Here's how the part is built. I have some questions about the finished solid (model axes, mm). Coordinates: 2 decimals unless noted, no trailing zeros. Write each loop counter-clockwise with the first axis right and the second up, starting at its lowest first coordinate (ties: lowest second). Pieces come first, ordered by that corner, then holes.
```python
from build123d import *

# Parameters (mm, degrees)
F0_W     = 53
F0_H     = 53
F0_R     = 1
F0_R_2   = 25.5
F1_DEPTH = 2
F2_SIZE  = 1.99999
F3_R     = 1


# Not quite as in the source:
# - a fillet or chamfer is up to 0.001 mm smaller than in the source, because OpenCascade refuses the exact size


with BuildPart() as f1:
    # F0 (on Top) → F1 (new body)
    with BuildSketch(Plane.XY):
        Rectangle(F0_W, F0_H)
        with Locations((-21.2132034356, -21.2132034356)):
            Circle(F0_R, mode=Mode.SUBTRACT)
        with Locations((21.2132034356, -21.2132034356)):
            Circle(F0_R, mode=Mode.SUBTRACT)
        with Locations((-21.2132034356, 21.2132034356)):
            Circle(F0_R, mode=Mode.SUBTRACT)
        Circle(F0_R_2, mode=Mode.SUBTRACT)
        with Locations((21.2132034356, 21.2132034356)):
            Circle(F0_R, mode=Mode.SUBTRACT)
    extrude(amount=F1_DEPTH)

    # F2 (size 2 in the source; OpenCascade refuses exactly that, so slightly less here)
    f2_edges = [f1.edges().sort_by_distance(p)[0] for p in [
        (-22.213203, 21.213203, 2),
        (20.213203, 21.213203, 2),
        (20.213203, -21.213203, 2),
        (-22.213203, -21.213203, 2),
    ]]
    chamfer(f2_edges, length=F2_SIZE)

    # F3
    f3_edges = [f1.edges().sort_by_distance(p)[0] for p in [
        (26.5, -26.5, 1),
        (26.5, 26.5, 1),
        (-26.5, -26.5, 1),
        (-26.5, 26.5, 1),
    ]]
    fillet(f3_edges, radius=F3_R)


solid = f1.part
```
1) We'd pull the mould along X, two halves only. Please class faces 1 (the face through (-5.5, -24.9, 1)), 2 (the face through (-26.5, 0, 1)), 3 (the face through (0, 26.5, 1)): pulls with the +X half, pulls with the -X half, needs draft (parallel to the pull), parting line crosses it, or undercut.
Values follow:
face 1: undercut
face 2: pulls with the -X half
face 3: needs draft
2) Imagine slicing it at C-C on z = 0.8. Please give me the cut outline in (x, y), then the cut area to 3 significant figures.
Values follow:
outline: (-26.5, -25.5) arc R1 ccw to (-25.5, -26.5) - (25.5, -26.5) arc R1 ccw to (26.5, -25.5) - (26.5, 25.5) arc R1 ccw to (25.5, 26.5) - (-25.5, 26.5) arc R1 ccw to (-26.5, 25.5) - close; hole circle Ø51 at (0, 0); hole circle Ø3.6 at (-21.21, -21.21); hole circle Ø3.6 at (-21.21, 21.21); hole circle Ø3.6 at (21.21, -21.21); hole circle Ø3.6 at (21.21, 21.21)
area: 725 mm2
3) Imagine slicing it at A-A on y = 0. Please give me the cut outline in (x, z).
Values follow:
outline: (-26.5, 0) - (-25.5, 0) - (-25.5, 2) - (-26.5, 2) - close; (25.5, 0) - (26.5, 0) - (26.5, 2) - (25.5, 2) - close
4) Will this pin go through, and if not, where does the flat tip stop? pin 1 (2.5 mm diameter, centred on x = 21.21, y = -21.21, fed in from +Z).
Values follow:
pin 1: stops at z = 0.25
5) I need wall thicknesses on probe 1 along Y at (x, z) = (-19, 1.85); probe 2 along Y at (x, z) = (23, 1.3) (3 decimals); probe 3 along Y at (x, z) = (12.5, 0.7). Which ranges of each line are inside material? Lowest first, please.
Values follow:
probe 1: y = -26.5 to -23.01, -19.42 to -17.01, 17.01 to 19.42, 23.01 to 26.5
probe 2: y = -26.5 to -22.661, -19.765 to -11.011, 11.011 to 19.765, 22.661 to 26.5
probe 3: y = -26.5 to -22.23, 22.23 to 26.5
6) Imagine slicing it at D-D on x = 21.5. Count the separate pieces of the cut face and the enclosed holes in it, then the cut area to 3 significant figures.
Values follow:
separate pieces: 4
enclosed holes: 0
area: 35.3 mm2
